Source: CAD feature listing. Evaluate the final solid. Frame: model axes, mm. Face numbers are marked on the shaded views. A direction names the side the tool comes from. Give positions to 0.01 mm unless a question says otherwise; leave off trailing zeros. Loops run counter-clockwise (first coordinate to the right, second up) from the corner with the lowest first, then second, coordinate; pieces in that order, holes last. Notation, with made-up numbers: M 35.5,-10 L 39.5,-10 A19 cw 39.5,11 Z; hole C 55,21.5 d2. An arc over 180 degrees is marked long. Put each result on its own line as item: value.
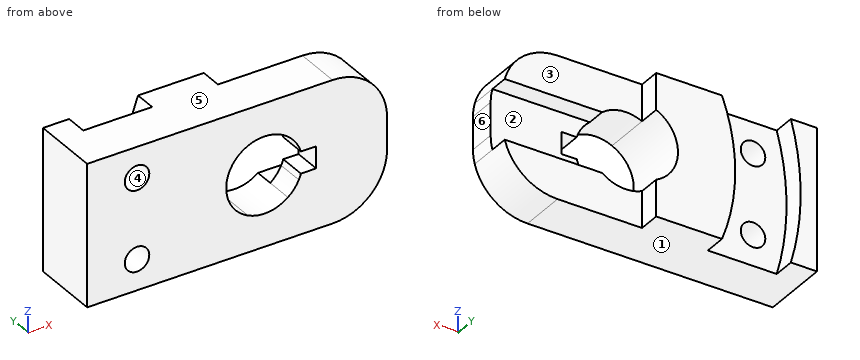
from build123d import *

# Parameters (mm, degrees)
BOSS_EXTRUDE1_DEPTH = 25
SKETCH1_3_R         = 4.5
BOSS_EXTRUDE2_DEPTH = 17
BOSS_EXTRUDE3_DEPTH = 25
BOSS_EXTRUDE4_DEPTH = 10


with BuildPart() as part:
    # Sketch1 → Boss-Extrude1 (new body)
    with BuildSketch(Plane(origin=(0, 0, 0), x_dir=(1, 0, 0), z_dir=(0, 1, 0))):
        with BuildLine():
            Line((0, 26), (0, -26))
            Line((0, -26), (9.587879583, -26))
            ThreePointArc((9.587879583, -26), (6, 0), (9.587879583, 26))
            Line((9.587879583, 26), (0, 26))
        make_face()
    extrude(amount=BOSS_EXTRUDE1_DEPTH)

    # Sketch1_3 → Boss-Extrude2 (add)
    # profile 1 of 4: a face of its own
    with BuildSketch(Plane(origin=(0, 0, 0), x_dir=(1, 0, 0), z_dir=(0, 1, 0))):
        with BuildLine():
            ThreePointArc((9.587879583, 26), (6, 0), (9.587879583, -26))
            Line((9.587879583, -26), (34.858358674, -26))
            ThreePointArc((34.858358674, -26), (30, 0), (34.858358674, 26))
            Line((34.858358674, 26), (9.587879583, 26))
        make_face()
        with Locations(Location((18.285849122, -14.728915195, 0), (0, 0, 270))):
            Circle(SKETCH1_3_R, mode=Mode.SUBTRACT)
        with Locations(Location((18.285849122, 14.728915195, 0), (0, 0, 270))):
            Circle(SKETCH1_3_R, mode=Mode.SUBTRACT)
    # profile 2 of 4: a face of its own
    with BuildSketch(Plane(origin=(0, 0, 0), x_dir=(1, 0, 0), z_dir=(0, 1, 0))):
        with BuildLine():
            Line((90, 26), (59, 26))
            Line((59, 26), (59, 12.649110641))
            ThreePointArc((59, 12.649110641), (66.564969445, 13.91225613), (73.660254038, 11))
            Line((73.660254038, 11), (109.364916731, 11))
            ThreePointArc((109.364916731, 11), (102.247448714, 21.811388301), (90, 26))
        make_face()
    # profile 3 of 4: a face of its own
    with BuildSketch(Plane(origin=(0, 0, 0), x_dir=(1, 0, 0), z_dir=(0, 1, 0))):
        with BuildLine():
            Line((59, -12.649110641), (59, -26))
            Line((59, -26), (90, -26))
            ThreePointArc((90, -26), (102.247448714, -21.811388301), (109.364916731, -11))
            Line((109.364916731, -11), (73.660254038, -11))
            ThreePointArc((73.660254038, -11), (66.564969445, -13.91225613), (59, -12.649110641))
        make_face()
    # profile 4 of 4: a face of its own
    with BuildSketch(Plane(origin=(0, 0, 0), x_dir=(1, 0, 0), z_dir=(0, 1, 0))):
        with BuildLine():
            ThreePointArc((34.858358674, 26), (30, 0), (34.858358674, -26))
            Line((34.858358674, -26), (59, -26))
            Line((59, -26), (59, -12.649110641))
            ThreePointArc((59, -12.649110641), (51, 0), (59, 12.649110641))
            Line((59, 12.649110641), (59, 26))
            Line((59, 26), (34.858358674, 26))
        make_face()
    extrude(amount=BOSS_EXTRUDE2_DEPTH)

    # Sketch1_4 → Boss-Extrude3 (add)
    with BuildSketch(Plane(origin=(0, 0, 0), x_dir=(1, 0, 0), z_dir=(0, 1, 0))):
        with BuildLine():
            ThreePointArc((34.858358674, 26), (30, 0), (34.858358674, -26))
            Line((34.858358674, -26), (59, -26))
            Line((59, -26), (59, -12.649110641))
            ThreePointArc((59, -12.649110641), (51, 0), (59, 12.649110641))
            Line((59, 12.649110641), (59, 26))
            Line((59, 26), (34.858358674, 26))
        make_face()
    extrude(amount=BOSS_EXTRUDE3_DEPTH)

    # Sketch1_5 → Boss-Extrude4 (add)
    with BuildSketch(Plane(origin=(0, 0, 0), x_dir=(1, 0, 0), z_dir=(0, 1, 0))):
        with BuildLine():
            Line((109.364916731, 11), (73.660254038, 11))
            ThreePointArc((73.660254038, 11), (75.944051158, 8.730850145), (77.649110641, 6))
            Line((77.649110641, 6), (110, 6))
            ThreePointArc((110, 6), (109.840593925, 8.52008585), (109.364916731, 11))
        make_face()
        with BuildLine():
            Line((73.660254038, -11), (109.364916731, -11))
            ThreePointArc((109.364916731, -11), (109.840593925, -8.52008585), (110, -6))
            Line((110, -6), (110, 6))
            Line((110, 6), (77.649110641, 6))
            ThreePointArc((77.649110641, 6), (78.071067812, 5.014697026), (78.416407865, 4))
            Line((78.416407865, 4), (84, 4))
            Line((84, 4), (84, -4))
            Line((84, -4), (78.416407865, -4))
            ThreePointArc((78.416407865, -4), (76.579928765, -7.86798893), (73.660254038, -11))
        make_face()
    extrude(amount=BOSS_EXTRUDE4_DEPTH)


solid = part.part
1. Contact query for flat-ended pins moving along their axis: P1, Ø14.5, axis at x = 19.5, z = 0.5, coming from the +Y side; P2, Ø2, axis at x = 99, y = 13, coming from the +Z side; P3, Ø7, axis at x = 18.29, z = -14.73, coming from the +Y side; P4, Ø6.5, axis at y = 20, z = 20.5, coming from the +X side. Output: stop coordinate, or through.
Found:
P1: y = 17
P2: z = 24.33
P3: through
P4: x = 104.98
2. Access query for the marked faces 1, 2 and 3. Directions: +Z, -Z, +X, -X, +Y, -Y. A direction counts if a zero-diameter tool reaches every point of the face in a straight line with its end or side. Return the directions, or none.
Found:
face 1: -Z, +X, -X, +Y, -Y
face 2: +X, +Y
face 3: +Z, -Z, +X, +Y
3. Section query C-C (x = 52.5). Output: boundary loops of the cut face in (y, z), plus the area to 3 significant figures.
Found:
outline: M 0,-26 L 25,-26 L 25,-6.3 L 0,-6.3 Z; M 0,6.3 L 25,6.3 L 25,26 L 0,26 Z
area: 985 mm^2
4. Material intervals for line 1 (X direction, y = 4.5, z = -12); line 2 (X direction, y = 16.5, z = 12.5); line 3 (Y direction, x = 26, z = -22.5), sorted ascending. Write a range as from..to.
Found:
line 1: 0..14.71, 21.86..57.79, 72.21..109.08
line 2: 0..14.38, 22.2..58.7, 71.3..108.91
line 3: 0..17
5. Section query D-D (y = 12.25). Output: boundary loops of the cut face in (x, z), plus the area to 3 significant figures.
Found:
outline: M 0,-26 L 90,-26 A20 ccw 109.36,-11 L 73.66,-11 A14 cw long 73.66,11 L 109.36,11 A20 ccw 90,26 L 0,26 Z; hole C 18.29,-14.73 d9; hole C 18.29,14.73 d9
area: 4,090 mm^2
6. Draft query along Z for the marked faces 4, 5 and 6. Return one class per face: pulls with the +Z half, pulls with the -Z half, needs draft (parallel to the pull), parting line crosses it, or undercut.
Found:
face 4: undercut
face 5: pulls with the +Z half
face 6: needs draft
7. Section query B-B (z = 0.5). Output: boundary loops of the cut face in (x, y), plus the area to 3 significant figures.
Found:
outline: M 0,0 L 51.01,0 L 51.01,25 L 30,25 L 30,17 L 6,17 L 6,25 L 0,25 Z; M 84,0 L 110,0 L 110,10 L 84,10 Z
area: 1,340 mm^2
8. Section query A-A (y = 18). Output: boundary loops of the cut face in (x, z), plus the area to 3 significant figures.
Found:
outline: M 0,-26 L 9.59,-26 A96 cw 9.59,26 L 0,26 Z; M 34.86,-26 L 59,-26 L 59,-12.65 A14 cw 59,12.65 L 59,26 L 34.86,26 A72 ccw Z
area: 1,650 mm^2
